from build123d import *

# Parameters (mm, degrees)
F0_W     = 102
F0_H     = 40
F0_W_2   = 240
F0_W_3   = 94
F0_H_2   = 25
F0_W_4   = 148
F0_W_5   = 92
F0_W_6   = 120
F0_H_3   = 19
F0_W_7   = 25
F0_H_4   = 92
F0_H_5   = 12
F0_W_8   = 12
F0_H_6   = 370
F0_W_9   = 87.5
F0_H_7   = 130
F0_W_10  = 212.5
F0_W_11  = 115
F0_W_12  = 150
F0_W_13  = 135.5
F1_DEPTH = 5
F2_DEPTH = 247
F3_W     = 40
F3_H     = 250
F3_W_2   = 102
F3_H_2   = 40
F3_W_3   = 240
F4_DEPTH = 40
F6_W     = 150
F6_H     = 40
F7_DEPTH = 150
F8_W     = 135.5
F8_H     = 40
F9_DEPTH = 60
F10_R    = 1


with BuildPart() as f1:
    # F0 (on Top) → F1 (new body)
    with BuildSketch(Plane.XY):
        Polygon((1170, -25), (1170, 820), (1042.5, 820), (1042.5, 780), (1130, 780), (1130, 622), (1130, 610), (1130, 15), (1090, 15), (1090, -25), align=None)
        with Locations((991.5, 800)):
            Rectangle(F0_W, F0_H)
        Polygon((940.5, 780), (940.5, 820), (725, 820), (725, 780), (787.5, 780), (812.5, 780), align=None)
        Polygon((15, 520), (-25, 520), (-25, 270), (15, 270), (15, 385), (15, 410), align=None)
        Polygon((458.5, -25), (685.5, -25), (685.5, 15), (572.5, 15), (560.5, 15), (470.5, 15), (458.5, 15), align=None)
        Polygon((685.5, -25), (787.5, -25), (787.5, 0), (787.5, 15), (685.5, 15), align=None)
        Polygon((787.5, -25), (850, -25), (850, 15), (812.5, 15), (787.5, 15), (787.5, 0), align=None)
        with Locations((970, -5)):
            Rectangle(F0_W_2, F0_H)
        Polygon((850, 15), (1090, 15), (1130, 15), (1130, 610), (1042.5, 610), (940.5, 610), (825.5, 610), (825.5, 549), (812.5, 549), (812.5, 237), (812.5, 145), (812.5, 15), align=None)
        with Locations((740.5, 397.5)):
            Rectangle(F0_W_3, F0_H_2)
        with Locations((301.5, 397.5)):
            Rectangle(F0_W_4, F0_H_2)
        with Locations((647.5, 397.5)):
            Rectangle(F0_W_5, F0_H_2)
        Polygon((601.5, 410), (507.5, 410), (495.5, 410), (495.5, 385), (601.5, 385), align=None)
        with Locations((435.5, 397.5)):
            Rectangle(F0_W_6, F0_H_2)
        Polygon((825.5, 691), (812.5, 691), (812.5, 549), (825.5, 549), (825.5, 610), (825.5, 622), align=None)
        with Locations((301.5, 419.5)):
            Rectangle(F0_W_4, F0_H_3)
        Polygon((495.5, 780), (331.5, 780), (181.5, 780), (15, 780), (15, 520), (15, 410), (227.5, 410), (227.5, 429), (375.5, 429), (375.5, 410), (495.5, 410), align=None)
        Polygon((1130, 780), (1042.5, 780), (940.5, 780), (812.5, 780), (812.5, 691), (825.5, 691), (825.5, 622), (940.5, 622), (1042.5, 622), (1130, 622), align=None)
        Polygon((311, 15), (323, 15), (323, 250.5), (328, 250.5), (328, 262.5), (311, 262.5), align=None)
        Polygon((572.5, 15), (685.5, 15), (787.5, 15), (787.5, 145), (787.5, 237), (787.5, 385), (693.5, 385), (601.5, 385), (495.5, 385), (375.5, 385), (227.5, 385), (15, 385), (15, 270), (15, 15), (88, 15), (238, 15), (311, 15), (311, 262.5), (328, 262.5), (328, 250.5), (323, 250.5), (323, 15), (458.5, 15), (458.5, 198.5), (450.5, 198.5), (450.5, 236.2157330513), (458.5, 236.2157330513), (458.5, 250.5), (420, 250.5), (420, 262.5), (470.5, 262.5), (470.5, 15), (560.5, 15), (560.5, 262.5), (685.5, 262.5), (685.5, 250.5), (572.5, 250.5), align=None)
        Polygon((812.5, 691), (812.5, 780), (787.5, 780), (787.5, 410), (787.5, 385), (787.5, 237), (812.5, 237), (812.5, 549), align=None)
        with Locations((800, 191)):
            Rectangle(F0_W_7, F0_H_4)
        with Locations((991.5, 616)):
            Rectangle(F0_W, F0_H_5)
        Polygon((560.5, 15), (572.5, 15), (572.5, 250.5), (685.5, 250.5), (685.5, 262.5), (560.5, 262.5), align=None)
        with Locations((501.5, 595)):
            Rectangle(F0_W_8, F0_H_6)
        with Locations((1086.25, 616)):
            Rectangle(F0_W_9, F0_H_5)
        with Locations((800, 80)):
            Rectangle(F0_W_7, F0_H_7)
        with Locations((121.25, 397.5)):
            Rectangle(F0_W_10, F0_H_2)
        Polygon((458.5, 198.5), (458.5, 15), (470.5, 15), (470.5, 262.5), (420, 262.5), (420, 250.5), (458.5, 250.5), (458.5, 236.2157330513), (450.5, 236.2157330513), (450.5, 198.5), align=None)
        with Locations((883, 616)):
            Rectangle(F0_W_11, F0_H_5)
        Polygon((787.5, 780), (725, 780), (575, 780), (507.5, 780), (507.5, 410), (601.5, 410), (693.5, 410), (787.5, 410), align=None)
        Polygon((181.5, 780), (181.5, 820), (-25, 820), (-25, 520), (15, 520), (15, 780), align=None)
        with Locations((256.5, 800)):
            Rectangle(F0_W_12, F0_H)
        Polygon((575, 780), (575, 820), (331.5, 820), (331.5, 780), (495.5, 780), (507.5, 780), align=None)
        with Locations((650, 800)):
            Rectangle(F0_W_12, F0_H)
        Polygon((15, 270), (-25, 270), (-25, -25), (88, -25), (88, 15), (15, 15), align=None)
        with Locations((163, -5)):
            Rectangle(F0_W_12, F0_H)
        Polygon((238, -25), (323, -25), (323, 15), (311, 15), (238, 15), align=None)
        with Locations((390.75, -5)):
            Rectangle(F0_W_13, F0_H)
    extrude(amount=F1_DEPTH)

    # F0 (on Top) → F2 (join)
    with BuildSketch(Plane.XY):
        Polygon((1170, -25), (1170, 820), (1042.5, 820), (1042.5, 780), (1130, 780), (1130, 622), (1130, 610), (1130, 15), (1090, 15), (1090, -25), align=None)
        Polygon((940.5, 780), (940.5, 820), (725, 820), (725, 780), (787.5, 780), (812.5, 780), align=None)
        Polygon((458.5, -25), (685.5, -25), (685.5, 15), (572.5, 15), (560.5, 15), (470.5, 15), (458.5, 15), align=None)
        Polygon((787.5, -25), (850, -25), (850, 15), (812.5, 15), (787.5, 15), (787.5, 0), align=None)
        with Locations((800, 80)):
            Rectangle(F0_W_7, F0_H_7)
        Polygon((812.5, 691), (812.5, 780), (787.5, 780), (787.5, 410), (787.5, 385), (787.5, 237), (812.5, 237), (812.5, 549), align=None)
        Polygon((825.5, 691), (812.5, 691), (812.5, 549), (825.5, 549), (825.5, 610), (825.5, 622), align=None)
        with Locations((883, 616)):
            Rectangle(F0_W_11, F0_H_5)
        with Locations((1086.25, 616)):
            Rectangle(F0_W_9, F0_H_5)
        with Locations((740.5, 397.5)):
            Rectangle(F0_W_3, F0_H_2)
        Polygon((601.5, 410), (507.5, 410), (495.5, 410), (495.5, 385), (601.5, 385), align=None)
        with Locations((501.5, 595)):
            Rectangle(F0_W_8, F0_H_6)
        with Locations((301.5, 419.5)):
            Rectangle(F0_W_4, F0_H_3)
        with Locations((301.5, 397.5)):
            Rectangle(F0_W_4, F0_H_2)
        Polygon((311, 15), (323, 15), (323, 250.5), (328, 250.5), (328, 262.5), (311, 262.5), align=None)
        Polygon((458.5, 198.5), (458.5, 15), (470.5, 15), (470.5, 262.5), (420, 262.5), (420, 250.5), (458.5, 250.5), (458.5, 236.2157330513), (450.5, 236.2157330513), (450.5, 198.5), align=None)
        Polygon((560.5, 15), (572.5, 15), (572.5, 250.5), (685.5, 250.5), (685.5, 262.5), (560.5, 262.5), align=None)
        Polygon((15, 270), (-25, 270), (-25, -25), (88, -25), (88, 15), (15, 15), align=None)
        Polygon((238, -25), (323, -25), (323, 15), (311, 15), (238, 15), align=None)
        with Locations((390.75, -5)):
            Rectangle(F0_W_13, F0_H)
        with Locations((163, -5)):
            Rectangle(F0_W_12, F0_H)
        Polygon((181.5, 780), (181.5, 820), (-25, 820), (-25, 520), (15, 520), (15, 780), align=None)
        with Locations((256.5, 800)):
            Rectangle(F0_W_12, F0_H)
        Polygon((575, 780), (575, 820), (331.5, 820), (331.5, 780), (495.5, 780), (507.5, 780), align=None)
        with Locations((650, 800)):
            Rectangle(F0_W_12, F0_H)
    extrude(amount=F2_DEPTH)

    # F3 (on face) → F4 (join)
    with BuildSketch(Plane.XY.offset(247)):
        with Locations((-5, 395)):
            Rectangle(F3_W, F3_H)
        with Locations((736.5, -5)):
            Rectangle(F3_W_2, F3_H_2)
        with Locations((970, -5)):
            Rectangle(F3_W_3, F3_H_2)
        with Locations((991.5, 800)):
            Rectangle(F3_W_2, F3_H_2)
    extrude(amount=-F4_DEPTH)

    # F6 (on offset) → F7 (cut)
    with BuildSketch(Plane.XY.offset(90)):
        with Locations((650, 800)):
            Rectangle(F6_W, F6_H)
        with Locations((256.5, 800)):
            Rectangle(F6_W, F6_H)
        with Locations((163, -5)):
            Rectangle(F6_W, F6_H)
    extrude(amount=F7_DEPTH, mode=Mode.SUBTRACT)

    # F8 (on face) → F9 (cut)
    with BuildSketch(Plane(origin=(0, 0, 240), x_dir=(1, 0, 0), z_dir=(0, 0, -1))):
        with Locations((390.75, 5)):
            Rectangle(F8_W, F8_H)
    extrude(amount=F9_DEPTH, mode=Mode.SUBTRACT)

    # F10
    f10_edges = [f1.edges().sort_by_distance(p)[0] for p in [
        (-25, -25, 123.5),
        (1170, -25, 123.5),
        (1170, 820, 123.5),
        (-25, 820, 123.5),
        (1130, 15, 126),
        (15, 15, 126),
        (15, 780, 126),
        (1130, 780, 126),
    ]]
    fillet(f10_edges, radius=F10_R)


solid = f1.part
Geometry check sheet. Reference: the model listing, model coordinates, mm. A direction names the side the tool comes from. Give positions to 0.01 mm unless a question says otherwise; leave off trailing zeros. Order: outer loops, then holes, each group sorted by start corner. A loop starts at its lowest first (then second) coordinate and runs counter-clockwise, first axis right, second up. Notation, with made-up numbers: M 57,58.25 L 113,58.25 A14 cw 113,79.25 Z; hole C -3.75,30 d3. An arc over 180 degrees is marked long. Use a Markdown table: item, result.
Item 1: Section check C-C (y = 166). Record the cut outline in (x, z), and give its area (3 significant figures).
Answers follow:
| item | result |
|---|---|
| outline | M -25,0 L 1170,0 L 1170,247 L 1130,247 L 1130,5 L 572.5,5 L 572.5,247 L 560.5,247 L 560.5,5 L 470.5,5 L 470.5,247 L 458.5,247 L 458.5,5 L 323,5 L 323,247 L 311,247 L 311,5 L 15,5 L 15,247 L -25,247 Z |
| area | 34,000 mm2 |
Item 2: Section check B-B (x = 1006.5). Record the cut outline in (y, z), and give its area (4 significant figures).
Answers follow:
| item | result |
|---|---|
| outline | M -25,0 L 820,0 L 820,5 L -25,5 Z; M -25,207 L 15,207 L 15,247 L -25,247 Z; M 780,207 L 820,207 L 820,247 L 780,247 Z |
| area | 7,425 mm2 |
Item 3: Section check D-D (z = 106). State how many separate pieces and enclosed holes the cut face has, and give its area (3 significant figures).
Answers follow:
| item | result |
|---|---|
| separate pieces | 8 |
| enclosed holes | 0 |
| area | 159,000 mm2 |
Item 4: Draft check along Y on faces 1 (the flat face through (300, 385, 124)), 2 (the flat face through (882, 610, 124)), 3 (the flat face through (991, 800, 207)). Enter one of: +Y half, -Y half, draft (parallel to the pull), parting line (faces both ways), or undercut.
Answers follow:
| item | result |
|---|---|
| face 1 | undercut |
| face 2 | undercut |
| face 3 | draft |
Item 5: Section check A-A (x = 357.5). Record the cut outline in (y, z), and give its area (3 significant figures).
Answers follow:
| item | result |
|---|---|
| outline | M -25,0 L 820,0 L 820,247 L 780,247 L 780,5 L 429,5 L 429,247 L 385,247 L 385,5 L 15,5 L 15,180 L -25,180 Z; M -25,240 L 15,240 L 15,247 L -25,247 Z |
| area | 31,800 mm2 |
Item 6: Depth check by flat-ended pin: P1, Ø12, axis at x = 434, y = 602, coming from the +Z side; P2, Ø7.5, axis at y = 402.5, z = 77, coming from the -X side; P3, Ø1.5, axis at x = 619.5, z = 195.5, coming from the +Y side. Enter the tip coordinate at first touch or a pass-through.
Answers follow:
| item | result |
|---|---|
| P1 | stops at z = 5 |
| P2 | stops at x = 227.5 |
| P3 | stops at y = 262.5 |
Item 7: Tool access check on faces 4 (the flat face through (1086, 610, 124)), 5 (the flat face through (649, 800, 240)), 6 (the flat face through (850, -5, 105)), 7 (the flat face through (564, 403, 0)). Record the directions out of +Z, -Z, +X, -X, +Y, -Y that give a thin tool (end or side, any length) a straight path to the whole face; none if there is none.
Answers follow:
| item | result |
|---|---|
| face 4 | +Z |
| face 5 | +Y |
| face 6 | -Y |
| face 7 | -Z, +X, -X, +Y, -Y |
Item 8: Material ranges on line 1 along X through (y, z) = (614, 198); line 2 along X through (y, z) = (521.5, 99); line 3 along X through (y, z) = (230.5, 139), recorded low to high.
Answers follow:
| item | result |
|---|---|
| line 1 | x = -25 to 15, 495.5 to 507.5, 787.5 to 940.5, 1042.5 to 1170 |
| line 2 | x = -25 to 15, 495.5 to 507.5, 787.5 to 812.5, 1130 to 1170 |
| line 3 | x = -25 to 15, 311 to 323, 450.5 to 470.5, 560.5 to 572.5, 1130 to 1170 |
